Could you check a few things on this model? Use its own coordinates, in mm. A direction names the side the tool comes from. Give positions to 0.01 mm unless a question says otherwise; leave off trailing zeros. Write each loop counter-clockwise with the first axis right and the second up, starting at its lowest first coordinate (ties: lowest second). Pieces come first, ordered by that corner, then holes. Notation, with made-up numbers: (80, 30) -> (129, 30) arc R15 cw to (129, 35) -> close; hole circle Ø7 at (6.5, 46). An arc over 180 degrees is marked (long way). One line per question, with ' | ' between items.
from build123d import *

# Parameters (mm, degrees)
BOSS_EXTRUDE2_DEPTH = 2
FILLET1_R           = 10
SKETCH3_R           = 7.2
SKETCH3_R_2         = 5.2
BOSS_EXTRUDE3_DEPTH = 2
SKETCH4_R           = 1.25
CUT_EXTRUDE1_DEPTH  = 2
SKETCH5_R           = 2
CUT_EXTRUDE2_DEPTH  = 1
SKETCH6_R           = 2.35
BOSS_EXTRUDE4_DEPTH = 5


with BuildPart() as part:
    # Sketch1 → Boss-Extrude2 (new body)
    with BuildSketch(Plane(origin=(0, 0, 0), x_dir=(1, 0, 0), z_dir=(0, 1, 0))):
        Polygon((-17.219288225, -19.914865419), (0.286329753, -19.914865419), (24.780711775, -9.023800613), (24.780711775, 13.326199387), (0.209283204, 24.085134581), (-17.219288225, 24.085134581), (-17.219288225, 12.085134581), (-21.219288225, 12.085134581), (-21.219288225, -7.914865419), (-17.219288225, -7.914865419), align=None)
    extrude(amount=BOSS_EXTRUDE2_DEPTH)

    # Fillet1
    # the kernel refuses this fillet: 10 mm, written as the material it adds along each edge
    with BuildSketch(Plane(origin=(-17.219288225, 0, 7.914865419), x_dir=(-1, 0, 0), z_dir=(0, 1, 0))) as fillet1_piece_1:
        with BuildLine():
            CenterArc((10, 8), FILLET1_R, 180, 53.130102354)
            Line((0, 8), (-0.2, 8))
            Line((-0.2, 8), (-0.2, 0))
            Line((-0.2, 0), (0, -0.2))
            ThreePointArc((0, -0.2), (2, -0.2), (3.88, -0.16))
            Line((3.88, -0.16), (4, 0))
        make_face()
    extrude(amount=2)
    with BuildSketch(Plane(origin=(-17.219288225, 0, -12.085134581), x_dir=(0, 0, -1), z_dir=(0, 1, 0))) as fillet1_piece_2:
        with BuildLine():
            CenterArc((8, 10), FILLET1_R, 216.869897646, 53.130102354)
            Line((0, 4), (-0.16, 3.88))
            ThreePointArc((-0.16, 3.88), (-0.2, 2), (-0.2, 0))
            Line((-0.2, 0), (0, -0.2))
            Line((0, -0.2), (8, -0.2))
            Line((8, -0.2), (8, 0))
        make_face()
    extrude(amount=2)

    # Sketch3 → Boss-Extrude3 (add)
    with BuildSketch(Plane(origin=(0, 2, 0), x_dir=(1, 0, 0), z_dir=(0, 1, 0))):
        with Locations(Location((11.568463112, 2.085134581, 0), (0, 0, 270))):
            Circle(SKETCH3_R)
        with Locations(Location((11.568463112, 2.085134581, 0), (0, 0, 270))):
            Circle(SKETCH3_R_2, mode=Mode.SUBTRACT)
    extrude(amount=BOSS_EXTRUDE3_DEPTH)

    # Sketch4 → Cut-Extrude1 (cut)
    with BuildSketch(Plane.XZ):
        with Locations(Location((11.568463112, -2.085134581, 0), (0, 0, 270))):
            Circle(SKETCH4_R)
    extrude(amount=-CUT_EXTRUDE1_DEPTH, mode=Mode.SUBTRACT)

    # Sketch5 → Cut-Extrude2 (cut)
    with BuildSketch(Plane.XZ):
        with Locations(Location((11.568463112, -2.085134581, 0), (0, 0, 270))):
            Circle(SKETCH5_R)
    extrude(amount=-CUT_EXTRUDE2_DEPTH, mode=Mode.SUBTRACT)

    # Sketch6 → Boss-Extrude4 (add)
    with BuildSketch(Plane(origin=(0, 2, 0), x_dir=(1, 0, 0), z_dir=(0, 1, 0))):
        with Locations(Location((19.780711775, -7.914865419, 0), (0, 0, 270))):
            Circle(SKETCH6_R)
        with Locations(Location((19.780711775, 12.085134581, 0), (0, 0, 270))):
            Circle(SKETCH6_R)
        with Locations(Location((-5.219288225, -7.914865419, 0), (0, 0, 270))):
            Circle(SKETCH6_R)
        with Locations(Location((-5.219288225, 12.085134581, 0), (0, 0, 270))):
            Circle(SKETCH6_R)
    extrude(amount=BOSS_EXTRUDE4_DEPTH)


solid = part.part
Q1. If we mould it in two halves opening along X, with no side actions, what happens to faces 4 (the cylindrical face through (18.707, 2.986, -3.022)), 5 (the flat face through (-5, 7, 8)), 6 (the cylindrical face through (13.55, 0.49, -1.82)), 7 (the flat face through (10, 1, -2))? For each: +X half, -X half, draft (parallel to the pull), parting line (faces both ways), or undercut.
Answer below:
face 4: parting line | face 5: draft | face 6: undercut | face 7: undercut
Q2. On a 3-axis mill with a long thin cutter (end or side, diameter ignored), from which of +Z, -Z, +X, -X, +Y, -Y can I reach the whole of each face in a straight line? I mean faces 1 (the flat face through (14, 4, 3)), 2 (the cylindrical face through (20.487, 4.465, 10.156)), 3 (the cylindrical face through (-18.246, 0.986, 11.501)). Say none if no direction works.
Answer below:
face 1: +X, -X, +Y | face 2: +Y | face 3: +Z, -X, +Y, -Y
Q3. Imagine slicing it at C-C on y = 5. Please give me the cut outline in (x, z), and give its area (3 significant figures).
Answer below:
outline: circle Ø4.7 at (-5.22, -12.09); circle Ø4.7 at (-5.22, 7.91); circle Ø4.7 at (19.78, -12.09); circle Ø4.7 at (19.78, 7.91) | area: 69.4 mm^2
Q4. If I drill on line 1 along Z through (x, y) = (20, 4.5); line 2 along Y through (x, z) = (5.5, 1); line 3 along Y through (x, z) = (14, -6), over which ranges is the centre line in solid material (lowest first)?
Answer below:
line 1: z = -14.42 to -9.75, 5.58 to 10.25 | line 2: y = 0 to 4 | line 3: y = 0 to 2
Q5. Imagine slicing it at A-A on z = 2.5. Please give me the cut outline in (x, y), and give its area (3 significant figures).
Answer below:
outline: (-21.22, 0) -> (24.78, 0) -> (24.78, 2) -> (17.12, 2) -> (17.12, 4) -> (14.02, 4) -> (14.02, 2) -> (9.12, 2) -> (9.12, 4) -> (6.02, 4) -> (6.02, 2) -> (-21.22, 2) -> close | area: 104 mm^2
Q6. Imagine slicing it at B-B on x = 9. Please give me the cut outline in (y, z), and give its area (3 significant figures).
Answer below:
outline: (0, -20.24) -> (2, -20.24) -> (2, -8.81) -> (4, -8.81) -> (4, -6.61) -> (2, -6.61) -> (2, 2.44) -> (4, 2.44) -> (4, 4.64) -> (2, 4.64) -> (2, 16.04) -> (0, 16.04) -> close | area: 81.4 mm^2
Q7. Will these pins go through, and if not, where does the flat tip stop? pin 1 (11.5 mm diameter, centred on x = 9, z = -4, fed in from +Y); pin 2 (8.5 mm diameter, centred on x = 11.57, z = -2.09, fed in from -Y); pin 3 (2 mm diameter, centred on x = 11.57, z = -2.09, fed in from -Y); pin 4 (5 mm diameter, centred on x = 4, z = 13, fed in from +Y).
Answer below:
pin 1: stops at y = 4 | pin 2: stops at y = 0 | pin 3: passes through | pin 4: stops at y = 2
Q8. Imagine slicing it at D-D on x = -13. Please give me the cut outline in (y, z), and give its area (3 significant figures).
Answer below:
outline: (0, -24.09) -> (2, -24.09) -> (2, 19.91) -> (0, 19.91) -> close | area: 88.0 mm^2
